```python
from build123d import *


with BuildPart() as part:
    # Sweep2: sweep along a path in Sketch1
    with BuildLine(Plane.XY) as sweep2_path:
        Line((0, 0), (-94.919661766, 0))
        ThreePointArc((-94.919661766, 0), (-98.455195672, 0.645856533), (-101.534040044, 2.5))
        ThreePointArc((-101.534040044, 2.5), (-109.841229183, -1.25), (-101.534040044, -5))
        ThreePointArc((-101.534040044, -5), (-98.455195672, -3.145856533), (-94.919661766, -2.5))
        Line((-94.919661766, -2.5), (0, -2.5))
    # Sketch2 → Sweep2 (sweep)
    with BuildSketch(Plane(origin=(0, 0, 0), x_dir=(0, 0, -1), z_dir=(1, 0, 0))):
        with BuildLine():
            Line((-1.25, 0), (1.25, 0))
            Line((1.25, 0), (1.485849057, 0.825471698))
            ThreePointArc((1.485849057, 0.825471698), (0, 3.5), (-1.485849057, 0.825471698))
            Line((-1.485849057, 0.825471698), (-1.25, 0))
        make_face()
    sweep(path=sweep2_path.line)


solid = part.part
```
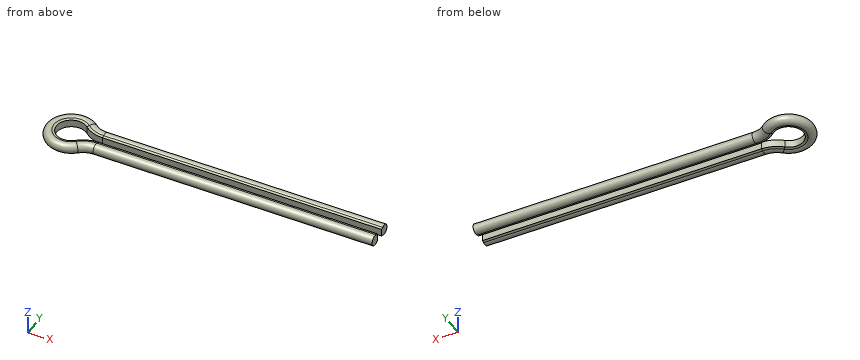
Input: part model. Units: mm. Frame: model coordinates. Coordinates: 2 decimals unless noted, no trailing zeros. Order: outer loops, then holes, each group sorted by start corner. A loop starts at its lowest first (then second) coordinate and runs counter-clockwise, first axis right, second up. Notation, with made-up numbers: (-26.75, -23) - (1.25, -23) arc R18 ccw to (1.25, -12) - close; hole circle Ø10 at (-19, 78.5). An arc over 180 degrees is marked (long way). Return JSON: item names as keys, results as strings.
Q1. First-contact query: pin 1 (1 mm diameter, centred on y = 0.5, z = -1, fed in from -X); pin 2 (2 mm diameter, centred on x = -51.5, z = -0.5, fed in from +Y); pin 3 (4 mm diameter, centred on x = -23.5, y = -6.5, fed in from -Z). Flat tips, straight axial feed; report the tip coordinate or a pass-through.
The answers:
{"pin 1": "stops at x = -113.11", "pin 2": "stops at y = 3.5", "pin 3": "stops at z = -1.73"}
Q2. Cut plane A-A (z = 0). Return loops of the section in (x, y) (3 decimals), then the cut area to 3 significant figures.
The answers:
{"outline": "(-101.534, -5) arc R5 cw (long way) to (-101.534, 2.5) arc R10 ccw to (-94.92, 0) - (0, 0) - (0, 3.5) - (-94.92, 3.5) arc R6.5 cw to (-99.219, 5.125) arc R8.5 ccw (long way) to (-99.219, -7.625) arc R6.5 cw to (-94.92, -6) - (0, -6) - (0, -2.5) - (-94.92, -2.5) arc R10 ccw to start", "area": "815 mm2"}
Q3. Ray query, probe 1 along Y at (x, z) = (-42, 0.2); probe 2 along X at (y, z) = (-5.25, -0.65); probe 3 along Y at (x, z) = (-53, -0.5). Return the intervals inside material, ascending.
The answers:
{"probe 1": "y = -5.99 to -2.5, 0 to 3.49", "probe 2": "x = -112.2 to -107.84, -101.84 to 0", "probe 3": "y = -5.93 to -2.5, 0 to 3.43"}
Q4. Cut plane B-B (x = -64). Return loops of the section in (y, z), then the cut area to 3 significant figures.
The answers:
{"outline": "(-3.33, -1.49) - (-2.5, -1.25) - (-2.5, 1.25) - (-3.33, 1.49) arc R1.75 ccw (long way) to start; (0, -1.25) - (0.83, -1.49) arc R1.75 ccw (long way) to (0.83, 1.49) - (0, 1.25) - close", "area": "20.3 mm2"}
Q5. Cut plane C-C (y = -1.25). Return loops of the section in (x, z).
The answers:
{"outline": "(-110.67, -1.49) - (-109.84, -1.25) - (-109.84, 1.25) - (-110.67, 1.49) arc R1.75 ccw (long way) to start"}
